For this review, take the finished solid that the model builds, in its own axes (mm). Face numbers are marked on the shaded views. Coordinates: 2 decimals unless noted, no trailing zeros. Write each loop counter-clockwise with the first axis right and the second up, starting at its lowest first coordinate (ties: lowest second). Pieces come first, ordered by that corner, then holes.
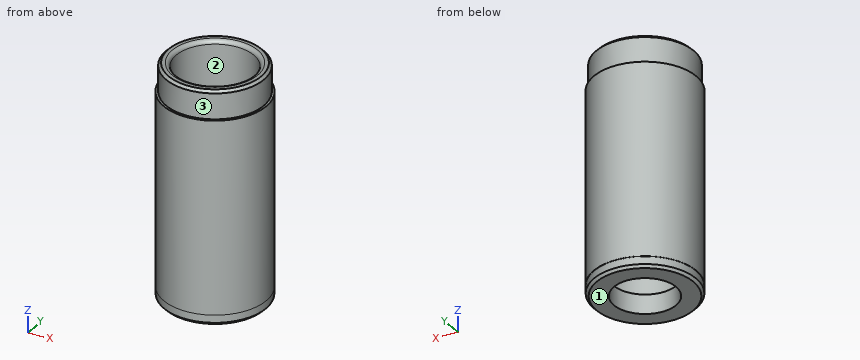
```python
from build123d import *

# Parameters (mm, degrees)
F2_R    = 1.5
F3_SIZE = 1


with BuildPart() as f1:
    # F0 (on Front) → F1 (revolve)
    with BuildSketch(Plane.XZ):
        Polygon((-15.15, -37.5), (-15.15, 45), (-19.075, 45), (-19.075, 34), (-19.975, 34), (-19.975, -41), (-19.9, -41), (-19.9, -45), (-12.15, -45), (-12.15, -37.5), align=None)
    revolve(axis=Axis((0, 0, -0.782523), (0, 0, -1)))

    # F2
    f2_edges = [f1.edges().sort_by_distance(p)[0] for p in [
        (15.15, 0, 45),
    ]]
    fillet(f2_edges, radius=F2_R)

    # F3
    f3_edges = [f1.edges().sort_by_distance(p)[0] for p in [
        (19.075, 0, 45),
        (19.9, 0, -45),
    ]]
    chamfer(f3_edges, length=F3_SIZE)


solid = f1.part
```
Q1. Add section C-C (z = 36). State the section outline as (x, y) points (3 decimals), then the cut area to 3 significant figures.
Ans:
outline: circle Ø38.15 at (0, 0); hole circle Ø30.3 at (0, 0)
area: 422 mm2
Q2. Draft analysis for pull direction X (two halves, no side actions). For the marked faces 1, 2 and 3, state which applies: +X half, -X half, draft (parallel to the pull), parting line (faces both ways), or undercut.
Ans:
face 1: draft
face 2: undercut
face 3: parting line
Q3. Add section A-A (y = 0). State the section outline as (x, z) points (3 decimals), then the cut area to 3 significant figures.
Ans:
outline: (-19.975, -41) - (-19.9, -41) - (-19.9, -44) - (-18.9, -45) - (-12.15, -45) - (-12.15, -37.5) - (-15.15, -37.5) - (-15.15, 43.5) arc R1.5 ccw to (-16.65, 45) - (-18.075, 45) - (-19.075, 44) - (-19.075, 34) - (-19.975, 34) - close; (12.15, -45) - (18.9, -45) - (19.9, -44) - (19.9, -41) - (19.975, -41) - (19.975, 34) - (19.075, 34) - (19.075, 44) - (18.075, 45) - (16.65, 45) arc R1.5 ccw to (15.15, 43.5) - (15.15, -37.5) - (12.15, -37.5) - close
area: 890 mm2
Q4. Clearance check with flat-ended pins moving along their axes: pin 1 Ø2 at (y, z) = (-3.5, -4.5) entering from -X; pin 2 Ø10 at (x, z) = (8, 5) entering from +Y; pin 3 Ø3 at (x, z) = (15.5, 14.5) entering from -Y; pin 4 Ø10 at (y, z) = (-3, 7.5) entering from +X (3 decimals). State where each tip first meets the part, or that it passes through.
Ans:
pin 1: stops at x = -19.82
pin 2: stops at y = 19.75
pin 3: stops at y = -14.25
pin 4: stops at x = 19.975
Q5. For probe 1 along Y at (x, z) = (0, -43); probe 2 along Y at (x, z) = (0, -27.5) (3 decimals); probe 3 along X at (y, z) = (0.5, -35), list the stretches that pass through material, from the lowest coordinate up.
Ans:
probe 1: y = -19.9 to -12.15, 12.15 to 19.9
probe 2: y = -19.975 to -15.15, 15.15 to 19.975
probe 3: x = -19.97 to -15.14, 15.14 to 19.97
Q6. Add section D-D (z = 18). State the section outline as (x, y) points (3 decimals), then the cut area to 3 significant figures.
Ans:
outline: circle Ø39.95 at (0, 0); hole circle Ø30.3 at (0, 0)
area: 532 mm2
